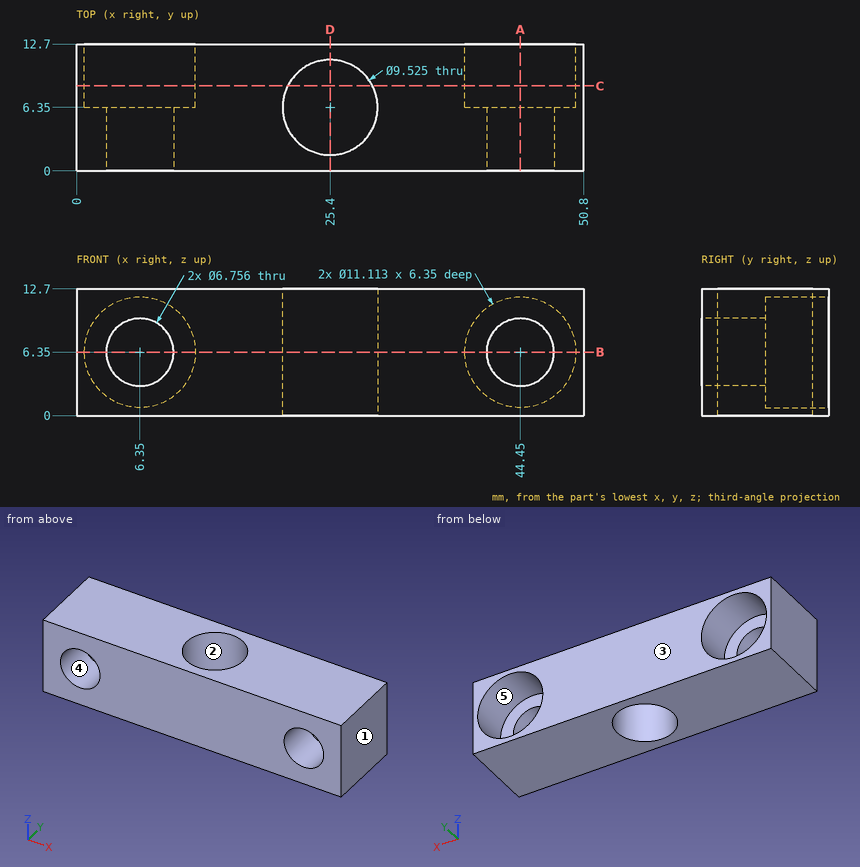
Check sheet for the drawn part. Datum: minimum x, y, z corner. Units: mm. A direction names the side the tool comes from. Give positions to 0.01 mm unless a question says otherwise; leave off trailing zeros. Order: outer loops, then holes, each group sorted by start corner. A loop starts at its lowest first (then second) coordinate and runs counter-clockwise, first axis right, second up. Notation, with made-up numbers: (16, -30.5) - (31, -30.5) arc R18 ccw to (31, -17.5) - close; hole circle Ø5 at (24, 30.5). An arc over 180 degrees is marked (long way). Write item = value, one per line. Start each with the question number.
1) Scan lines: L1, parallel to X at y = 12, z = 6.5 (1 decimal); L2, parallel to Z at x = 44.45, y = 2.5; L3, parallel to X at y = 6.5, z = 8.75. Record each from-to range of solid material in increasing order.
2) Section check D-D (x = 25.4). Enter the section's corners in (y, z).
3) Gauge pin test, flat ends, axial feed: pin 1 Ø6 at (x, z) = (6.35, 6.35) entering from +Y; pin 2 Ø3 at (x, y) = (7.5, 3) entering from -Z. Record the tip position at first contact, or that the pin passes through.
4) Draft check along X on the marked faces 1, 2 and 3. Enter one of: released by +X, released by -X, zero draft, split by the parting line, or undercut.
5) Access from +Z, -Z, +X, -X, +Y, -Y to the whole of each face (thin tool, end or side, straight path). Record for the marked faces 4 and 5.
6) Section check C-C (y = 8.5). Enter the section's corners in (x, z).
7) Section check B-B (z = 6.35). Count the separate pieces of the cut face and the enclosed holes in it, then the cut area to 3 significant figures.
8) Section check A-A (x = 44.45). Enter the section's corners in (y, z).
Geometry check:
q1.L1 = 0 to 0.8, 11.9 to 38.9, 50 to 50.8
q1.L2 = 0 to 2.97, 9.73 to 12.7
q1.L3 = 0 to 1.34, 11.36 to 20.64, 30.16 to 39.44, 49.46 to 50.8
q2.outline = (0, 0) - (1.59, 0) - (1.59, 12.7) - (0, 12.7) - close; (11.11, 0) - (12.7, 0) - (12.7, 12.7) - (11.11, 12.7) - close
q3.pin_1 = through
q3.pin_2 = 0
q4.face_1 = released by +X
q4.face_2 = undercut
q4.face_3 = zero draft
q5.face_4 = +Y, -Y
q5.face_5 = +Y
q6.outline = (0, 0) - (21.15, 0) - (21.15, 12.7) - (0, 12.7) - close; (29.65, 0) - (50.8, 0) - (50.8, 12.7) - (29.65, 12.7) - close; hole circle Ø11.11 at (6.35, 6.35); hole circle Ø11.11 at (44.45, 6.35)
q7.separate_pieces = 3
q7.enclosed_holes = 1
q7.area = 347 mm2
q8.outline = (0, 0) - (12.7, 0) - (12.7, 0.79) - (6.35, 0.79) - (6.35, 2.97) - (0, 2.97) - close; (0, 9.73) - (6.35, 9.73) - (6.35, 11.91) - (12.7, 11.91) - (12.7, 12.7) - (0, 12.7) - close
